Work out the finished part from the listing and answer in its coordinate system (mm). A direction names the side the tool comes from. Coordinates: 2 decimals unless noted, no trailing zeros. Loops run counter-clockwise (first coordinate to the right, second up) from the corner with the lowest first, then second, coordinate; pieces in that order, holes last. Notation, with made-up numbers: (-30.5, 34.5) -> (-6.5, 34.5) arc R29 cw to (-6.5, 73.5) -> close; hole circle Ø8 at (4.5, -7.75). An arc over 180 degrees is marked (long way). Use a Markdown table: item, result.
from build123d import *

# Parameters (mm, degrees)
F0_W     = 100
F0_H     = 100
F1_DEPTH = 100
F2_R     = 35
F3_DEPTH = 70
F4_R     = 35
F5_DEPTH = 70
F7_D     = 5


with BuildPart() as f1:
    # F0 (on Front) → F1 (new body)
    with BuildSketch(Plane.XZ):
        with Locations((50, 50)):
            Rectangle(F0_W, F0_H)
    extrude(amount=F1_DEPTH)

    # F2 (on face) → F3 (join)
    with BuildSketch(Plane.XY.offset(100)):
        with Locations((47.518581, -50.615475)):
            Circle(F2_R)
    extrude(amount=F3_DEPTH)

    # F4 (on face) → F5 (join)
    with BuildSketch(Plane(origin=(0, 0, 0), x_dir=(1, 0, 0), z_dir=(0, 0, -1))):
        with Locations((49.175262, 49.722657)):
            Circle(F4_R)
    extrude(amount=F5_DEPTH)

    # F7 (through all)
    with Locations(Plane.YZ.offset(100)):
        with Locations((-53.554386, 50)):
            Hole(F7_D / 2)


solid = f1.part
Q1. Section A-A on z = 50 is taken. Determine the outline of the cut face in (x, y), and give its area (3 significant figures).
Solved:
| item | result |
|---|---|
| outline | (0, -100) -> (100, -100) -> (100, -56.05) -> (0, -56.05) -> close; (0, -51.05) -> (100, -51.05) -> (100, 0) -> (0, 0) -> close |
| area | 9,500 mm² |
Q2. Section C-C on y = -27.5 is taken. Determine the outline of the cut face in (x, z), and give its area (3 significant figures).
Solved:
| item | result |
|---|---|
| outline | (0, 0) -> (22.14, 0) -> (22.14, -70) -> (76.22, -70) -> (76.22, 0) -> (100, 0) -> (100, 100) -> (73.8, 100) -> (73.8, 170) -> (21.24, 170) -> (21.24, 100) -> (0, 100) -> close |
| area | 17,500 mm² |
Q3. Section B-B on x = 52.5 is taken. Determine the outline of the cut face in (y, z).
Solved:
| item | result |
|---|---|
| outline | (-100, 0) -> (-84.56, 0) -> (-84.56, -70) -> (-14.88, -70) -> (-14.88, 0) -> (0, 0) -> (0, 100) -> (-15.97, 100) -> (-15.97, 170) -> (-85.26, 170) -> (-85.26, 100) -> (-100, 100) -> close; hole circle Ø5 at (-53.55, 50) |
Q4. Section D-D on x = 87 is taken. Determine the outline of the cut face in (y, z), and give its area (3 significant figures).
Solved:
| item | result |
|---|---|
| outline | (-100, 0) -> (0, 0) -> (0, 100) -> (-100, 100) -> close; hole circle Ø5 at (-53.55, 50) |
| area | 9,980 mm² |
Q5. Consider line 1 (Y direction, x = 47.5, z = 141.5); line 2 (Z direction, x = 8, y = -77); line 3 (Y direction, x = 50.5, z = -12.5). Determine where each line is inside the solid, lowest interval first. Write a range as [from, to].
Solved:
| item | result |
|---|---|
| line 1 | [-85.62, -15.62] |
| line 2 | [0, 100] |
| line 3 | [-84.7, -14.75] |
Q6. Given pin 1 Ø12 at (y, z) = (-29.5, -33.5) entering from +X; pin 2 Ø8 at (x, z) = (65, -27) entering from -Y; pin 3 Ø6 at (y, z) = (-76, 127) entering from +X, each flat-ended and moving along its own axis, determine where each tip first touches the part or whether it passes through.
Solved:
| item | result |
|---|---|
| pin 1 | x = 81.16 |
| pin 2 | y = -82.66 |
| pin 3 | x = 74.42 |
Q7. Determine the mould class of faces 4 (the cylindrical face through (49.3, -51.057, 50.11)), 5 (the flat face through (47, -50, 170)), 6 (the cylindrical face through (80.9, -40.1, 134.5)), 7 (the flat face through (49, -50, -70)) for opening direction Z: pulls with the +Z half, pulls with the -Z half, needs draft (parallel to the pull), parting line crosses it, or undercut.
Solved:
| item | result |
|---|---|
| face 4 | undercut |
| face 5 | pulls with the +Z half |
| face 6 | needs draft |
| face 7 | pulls with the -Z half |
Q8. For faces 1 (the flat face through (83, -49, 100)), 2 (the flat face through (49, 0, 51)), 3 (the cylindrical face through (65.326, -18.672, -34.51)), determine the directions among +Z, -Z, +X, -X, +Y, -Y from which every point of the face is accessible in a straight line to the end or side of a thin tool.
Solved:
| item | result |
|---|---|
| face 1 | +Z |
| face 2 | +Z, -Z, +X, -X, +Y |
| face 3 | -Z |
